from build123d import *

# Parameters (mm, degrees)
BOSS_EXTRUDE2_DEPTH      = 152.4
BOSS_EXTRUDE2_DEPTH_BACK = 152.4
BOSS_EXTRUDE3_DEPTH      = 46.228


with BuildPart() as part:
    # Sketch3 → Boss-Extrude2 (new, two sides: drawn at the far end of the back side and taken through both)
    with BuildSketch(Plane.XY.offset(-BOSS_EXTRUDE2_DEPTH_BACK)):
        Polygon((-6.35, -3.666174209), (0, -7.332348419), (6.35, -3.666174209), (6.35, 3.666174209), (0, 7.332348419), (-6.35, 3.666174209), align=None)
    extrude(amount=BOSS_EXTRUDE2_DEPTH + BOSS_EXTRUDE2_DEPTH_BACK)

    # Sketch4 → Boss-Extrude3 (add)
    with BuildSketch(Plane.XY.offset(152.4)):
        Polygon((-6.35, 3.666174209), (-6.35, -3.666174209), (0, -7.332348419), (6.35, -3.666174209), (6.35, 3.666174209), (0, 7.332348419), align=None)
    extrude(amount=BOSS_EXTRUDE3_DEPTH)


solid = part.part
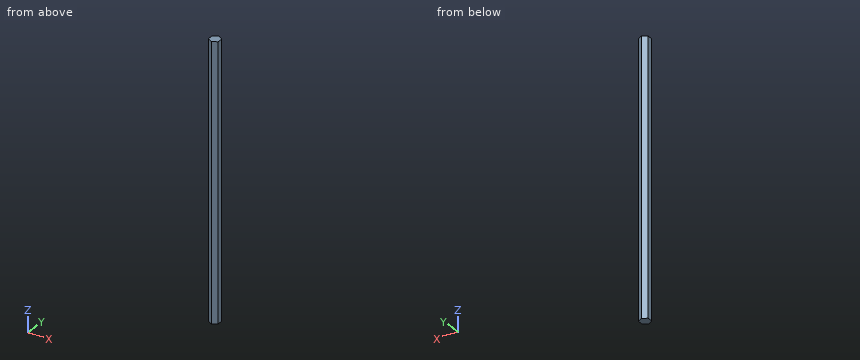
Can you work these out from the model? Positions are in its coordinate system, mm. Give positions to 0.01 mm unless a question says otherwise; leave off trailing zeros. Order: outer loops, then holes, each group sorted by start corner. A loop starts at its lowest first (then second) coordinate and runs counter-clockwise, first axis right, second up. Notation, with made-up numbers: M 35,38 L 63,38 A25 cw 63,72 Z; hole C 52,15.25 d11. An arc over 180 degrees is marked long. Use a Markdown table: item, result. Add a question column.
Item 1: Suppose I cut it at A-A (z = 6.5). List the corners of the cut face in (x, y) for me, then the cut area to 3 significant figures.
Item 2: If I drill on L1, parallel to Y at x = 6.25, z = 160; L2, parallel to X at y = -5.25, z = 171; L3, parallel to Y at x = 1.75, z = 130, over which ranges is the centre line in solid material (lowest first)? Write a range as [from, to].
Item 3: Suppose I cut it at B-B (x = 3). List the corners of the cut face in (y, z) for me.
Item 4: Will these pins go through, and if not, where does the flat tip stop? pin 1 (2 mm diameter, centred on x = 1.5, z = 10.5, fed in from -Y); pin 2 (6 mm diameter, centred on x = -1.5, z = -43.5, fed in from +Y).
Answer sheet:
| question | item | result |
|---|---|---|
| 1 | outline | M -6.35,-3.67 L 0,-7.33 L 6.35,-3.67 L 6.35,3.67 L 0,7.33 L -6.35,3.67 Z |
| 1 | area | 140 mm² |
| 2 | L1 | y = [-3.72, 3.72] |
| 2 | L2 | x = [-3.61, 3.61] |
| 2 | L3 | y = [-6.32, 6.32] |
| 3 | outline | M -5.6,-152.4 L 5.6,-152.4 L 5.6,198.63 L -5.6,198.63 Z |
| 4 | pin 1 | stops at y = -7.04 |
| 4 | pin 2 | stops at y = 7.33 |
